Autodesk Inventor part; units mm, degrees
ref_plane "YZ Plane" through (0, 0, 0) normal (1, 0, 0) x (0, 1, 0)
ref_plane "XZ Plane" through (0, 0, 0) normal (0, 1, 0) x (-1, 0, 0)
ref_plane "XY Plane" through (0, 0, 0) normal (0, 0, 1) x (1, 0, 0)
sketch "Sketch1" plane through (0, 0, 0) normal (0, 1, 0) x (-1, 0, 0)
  circle A0 centre (0, 0) radius 22.5
  circle A1 centre (0, 0) radius 37.5
  dimension "d0" = 45
  dimension "d1" = 75
extrude "Extrusion1" add sketch "Sketch1" along normal blind 2
sketch "Sketch2" plane through (0, 2, 0) normal (0, 1, 0) x (1, 0, 0)
  circle A0 centre (0, 0) radius 37.5
  circle A1 centre (0, 0) radius 22.5
  circle A2 centre (0, 0) radius 32.4
  dimension "d4" = 64.8
extrude "Extrusion2" add sketch "Sketch2" along normal blind 12.7 contours A2
feature "FaceDraft1" [suppressed]
sketch "Sketch3" plane through (0, 14.7, 0) normal (0, 1, 0) x (1, 0, 0)
  circle A0 centre (26.4608, -5.3692) radius 2.875
  circle A1 centre (17.8802, 20.2311) radius 2.875
  circle A2 centre (-8.5805, 25.6003) radius 2.875
  circle A3 centre (-26.4608, 5.3692) radius 2.875
  circle A4 centre (-17.8802, -20.2311) radius 2.875
  circle A5 centre (8.5805, -25.6003) radius 2.875
  point P0 (0, 0)
extrude "Extrusion3" cut sketch "Sketch3" against normal through all
sketch "Sketch4" plane through (0, 0, 0) normal (0, -1, 0) x (1, 0, 0)
  circle A0 centre (26.4608, 5.3692) radius 2.875
  line L0 (30.7783, 3.7285) -> (27.1986, 0.8097)
  line L1 (27.1986, 0.8097) -> (22.8811, 2.4504)
  line L2 (22.8811, 2.4504) -> (22.1432, 7.0099)
  line L3 (22.1432, 7.0099) -> (25.7229, 9.9287)
  line L4 (25.7229, 9.9287) -> (30.0404, 8.2879)
  line L5 (30.0404, 8.2879) -> (30.7783, 3.7285)
  point P0 (0, 0)
  dimension "d10" = 8
extrude "Extrusion4" cut sketch "Sketch4" against normal blind 5 contours A0 | L0 L1 L2 L3 L4 L5
pattern_circular "Circular Pattern1" count 6 over 360 about axis through (0, 2, 0) along (0, 1, 0) of "Extrusion4"
properties part number "j1Flange"
The model under review builds one solid part; all positions refer to its coordinate system, in mm. A direction names the side the tool comes from. Coordinates: 2 decimals unless noted, no trailing zeros. Loops run counter-clockwise (first coordinate to the right, second up) from the corner with the lowest first, then second, coordinate; pieces in that order, holes last.
(1) Draft analysis for pull direction Z (two halves, no side actions). For faces 3 (the cylindrical face through (4.88, 0.99, -37.18)), 4 (the flat face through (6.03, 2.46, 28.68)), state which applies: +Z half, -Z half, draft (parallel to the pull), parting line (faces both ways), or undercut.
Determined:
face 3: parting line
face 4: undercut
(2) Consider section A-A, the plane y = 8.25. Give the number of separate pieces and of enclosed holes in the cut face, plus the area to 3 significant figures.
Determined:
separate pieces: 1
enclosed holes: 7
area: 1,550 mm2
(3) Wall thickness on L1, parallel to Z at x = -10, y = 11; L2, parallel to X at y = 8.25, z = -4.5; L3, parallel to X at y = 13.5, z = 18.5: over which ranges is each line inside the solid? List them lowest first.
Determined:
L1: z = -30.82 to -28.1, -23.1 to -20.16, 20.16 to 30.82
L2: x = -32.09 to -29.2, -23.72 to -22.05, 22.05 to 32.09
L3: x = -26.6 to -20.18, -15.58 to -12.81, 12.81 to 26.6
(4) Tool access review of faces 1 (the flat face through (-4.637, 2.465, -24.929)), 2 (the cylindrical face through (-27.08, 9.92, -2.56)): name each direction out of +Z, -Z, +X, -X, +Y, -Y from which nothing blocks a thin tool from reaching the whole face with its end or side.
Determined:
face 1: -Y
face 2: +Y, -Y
(5) Consider section C-C, the plane z = 31.5. Give the boundary of the cut face in (x, y), plus the area to 3 significant figures.
Determined:
outline: (-20.35, 0) - (20.35, 0) - (20.35, 2) - (7.58, 2) - (7.58, 14.7) - (-7.58, 14.7) - (-7.58, 2) - (-20.35, 2) - close
area: 274 mm2
(6) Insertion check: P1, Ø5, axis at x = -8.58, z = -25.6, coming from the -Y side; P2, Ø1.5, axis at x = 11.5, y = 11.5, coming from the -Z side; P3, Ø5, axis at x = 29.5, y = 9.5, coming from the +Z side; P4, Ø6, axis at y = 13, z = -27, coming from the -X side. Each pin has a flat end and moves straight along its axis. Give the tip position at first contact, or say it passes through.
Determined:
P1: passes through
P2: stops at z = -30.56
P3: stops at z = 17.91
P4: stops at x = -21.77
